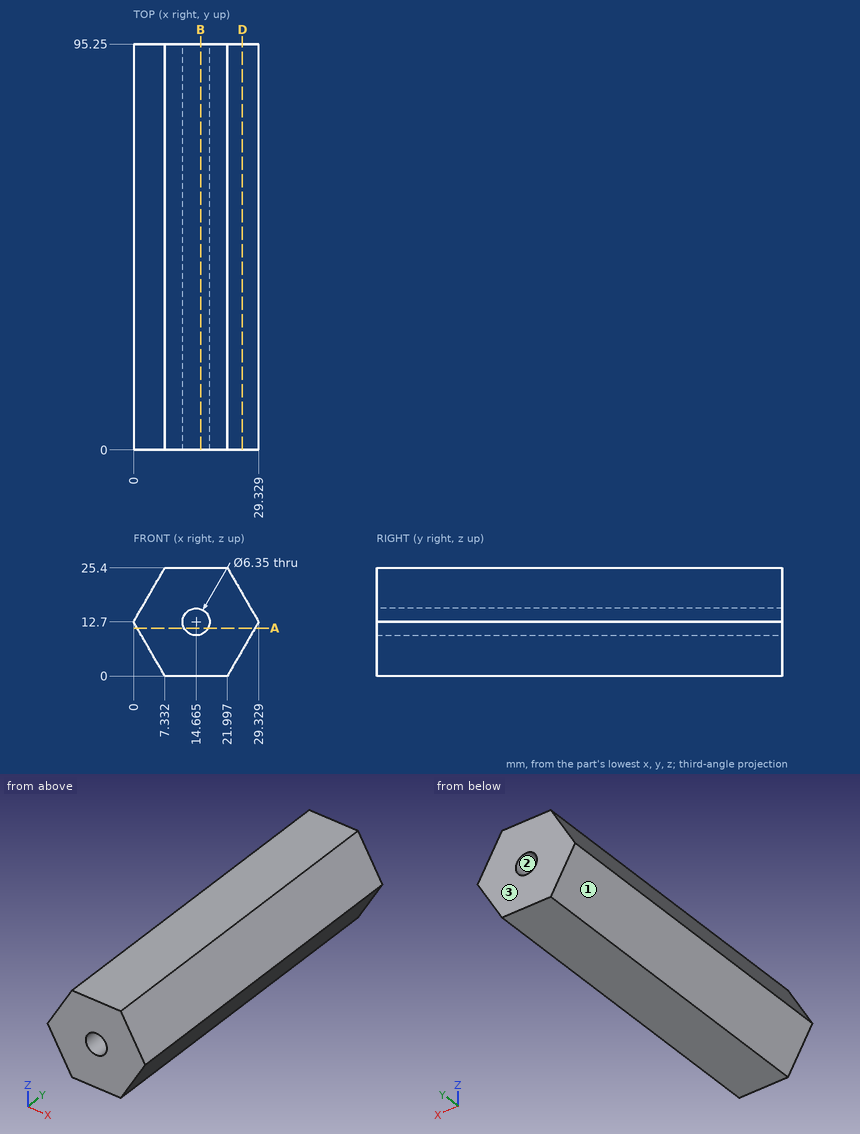
Study the drawing (mm; zero at the part's minimum x, y, z) and answer. Round coordinates to 2 decimals unless told otherwise and drop trailing zeros. Write each loop counter-clockwise with the first axis right and the second up, starting at its lowest first coordinate (ties: lowest second). Pieces come first, ordered by that corner, then holes.
1) A cutting plane is placed at D-D on x = 25.5. Determine the outline of the cut face in (y, z).
2) Flat-ended cylindrical pins translate along their axes: P1, Ø4, axis at y = 16, z = 19.5, coming from the +X side; P2, Ø4, axis at x = 14.66, z = 12.7, coming from the +Y side; P3, Ø6, axis at y = 30.5, z = 18, coming from the +X side. Find the tip coordinate at first contact, or state that the pin passes through.
3) A cutting plane is placed at B-B on x = 15.75. Determine the outline of the cut face in (y, z).
4) Determine the mould class of the marked faces 1, 2 and 3 for opening direction X: pulls with the +X half, pulls with the -X half, needs draft (parallel to the pull), parting line crosses it, or undercut.
5) A cutting plane is placed at A-A on z = 11.25. Determine the outline of the cut face in (x, y).
6) Consider probe 1 along X at (y, z) = (76, 12.7); probe 2 along Z at (x, y) = (16.5, 41); probe 3 along X at (y, z) = (6.5, 15.25) (1 decimal). Determine where each line is inside the solid, lowest interval first.
Entries:
1. outline: (0, 6.07) - (95.25, 6.07) - (95.25, 19.33) - (0, 19.33) - close
2. P1: stops at x = 26.56
2. P2: passes through
2. P3: stops at x = 28
3. outline: (0, 0) - (95.25, 0) - (95.25, 9.72) - (0, 9.72) - close; (0, 15.68) - (95.25, 15.68) - (95.25, 25.4) - (0, 25.4) - close
4. face 1: pulls with the -X half
4. face 2: undercut
4. face 3: needs draft
5. outline: (0.84, 0) - (11.84, 0) - (11.84, 95.25) - (0.84, 95.25) - close; (17.49, 0) - (28.49, 0) - (28.49, 95.25) - (17.49, 95.25) - close
6. probe 1: x = 0 to 11.49, 17.84 to 29.33
6. probe 2: z = 0 to 10.11, 15.29 to 25.4
6. probe 3: x = 1.5 to 12.8, 16.6 to 27.9
